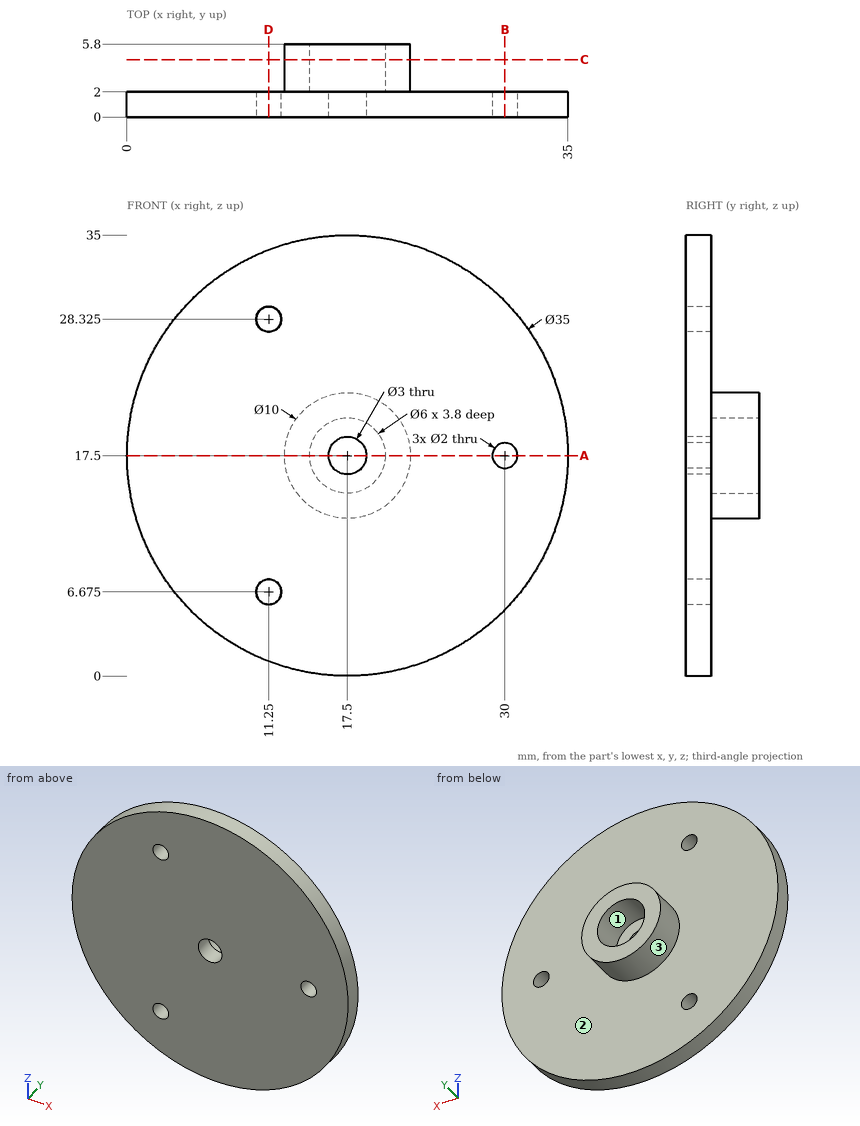
Job drawing, mm, ordinate dimensions from the low corner. One solid piece. Coordinates: 2 decimals unless noted, no trailing zeros. Write each loop counter-clockwise with the first axis right and the second up, starting at its lowest first coordinate (ties: lowest second). Pieces come first, ordered by that corner, then holes. Notation, with made-up numbers: (68, 21) - (89, 21) arc R28 cw to (89, 50) - close; hole circle Ø11 at (-2, -4). An arc over 180 degrees is marked (long way). Use a Markdown table: item, result. Add a question column.
Item 1: Band-saw the part on C-C, the plane y = 4.55. Give the cut face in (x, z).
Item 2: Band-saw the part on B-B, the plane x = 30. Give the cut face in (y, z).
Item 3: Mould opens along X. For the marked faces 1, 2 and 3 say: pulls with the +X half, pulls with the -X half, needs draft (parallel to the pull), parting line crosses it, or undercut.
Item 4: Flat gauge pins, fed straight in: pin 1 (4 mm diameter, centred on x = 17.5, z = 17.5, fed in from +Y); pin 2 (1.8 mm diameter, centred on x = 30, z = 17.5, fed in from +Y); pin 3 (1 mm diameter, centred on y = 1.5, z = 10, fed in from -X); pin 4 (2 mm diameter, centred on y = 0.5, z = 13, fed in from +X). Where does each tip first touch, or does it go through?
Item 5: Drill centre lines: L1, parallel to Z at x = 17.5, y = 0.8; L2, parallel to Z at x = 11.25, y = 0.8 (1 decimal); L3, parallel to Y at x = 16, z = 30.5. Where is each one in solid material? Low to high. Write a range as from..to.
Item 6: Band-saw the part on A-A, the plane z = 17.5. Give the cut face in (x, y).
Item 7: Band-saw the part on D-D, the plane x = 11.25. Give the cut face in (y, z) (1 decimal).
Numbers:
| question | item | result |
|---|---|---|
| 1 | outline | circle Ø10 at (17.5, 17.5); hole circle Ø6 at (17.5, 17.5) |
| 2 | outline | (0, 5.25) - (2, 5.25) - (2, 16.5) - (0, 16.5) - close; (0, 18.5) - (2, 18.5) - (2, 29.75) - (0, 29.75) - close |
| 3 | face 1 | undercut |
| 3 | face 2 | needs draft |
| 3 | face 3 | parting line crosses it |
| 4 | pin 1 | y = 2 |
| 4 | pin 2 | through |
| 4 | pin 3 | x = 1.46 |
| 4 | pin 4 | x = 34.65 |
| 5 | L1 | 0..16, 19..35 |
| 5 | L2 | 1.2..5.7, 7.7..27.3, 29.3..33.8 |
| 5 | L3 | 0..2 |
| 6 | outline | (0, 0) - (16, 0) - (16, 2) - (14.5, 2) - (14.5, 5.8) - (12.5, 5.8) - (12.5, 2) - (0, 2) - close; (19, 0) - (29, 0) - (29, 2) - (22.5, 2) - (22.5, 5.8) - (20.5, 5.8) - (20.5, 2) - (19, 2) - close; (31, 0) - (35, 0) - (35, 2) - (31, 2) - close |
| 7 | outline | (0, 1.2) - (2, 1.2) - (2, 5.7) - (0, 5.7) - close; (0, 7.7) - (2, 7.7) - (2, 27.3) - (0, 27.3) - close; (0, 29.3) - (2, 29.3) - (2, 33.8) - (0, 33.8) - close |
